Geometry: final body of the model. Coordinates: model frame, mm. Give positions to 0.01 mm unless a question says otherwise; leave off trailing zeros. Write each loop counter-clockwise with the first axis right and the second up, starting at its lowest first coordinate (ties: lowest second). Pieces come first, ordered by that corner, then holes. Notation, with made-up numbers: M -18,-17 L 30,-17 A28 cw 30,20 Z; hole C -2.5,0 d9. An arc over 180 degrees is marked long. Use a Markdown table: item, result. Add a question column.
(1) Cut plane B-B (x = -423.5). Output: boundary loops of the cut face in (y, z).
(2) Cut plane A-A (y = -565). Output: boundary loops of the cut face in (x, z).
(3) Pin query (flat end, axial travel): pin 1 Ø14 at (y, z) = (-533, 39.5) entering from +X; pin 2 Ø10 at (x, z) = (554, 38) entering from +Y; pin 3 Ø6.5 at (x, z) = (-301.5, 7.5) entering from -Y. Return the tip coordinate at first contact, or that it passes through.
(4) Material intervals for L1, parallel to Y at x = 155, z = 35; L2, parallel to X at y = -472, z = 11.5, sorted ascending.
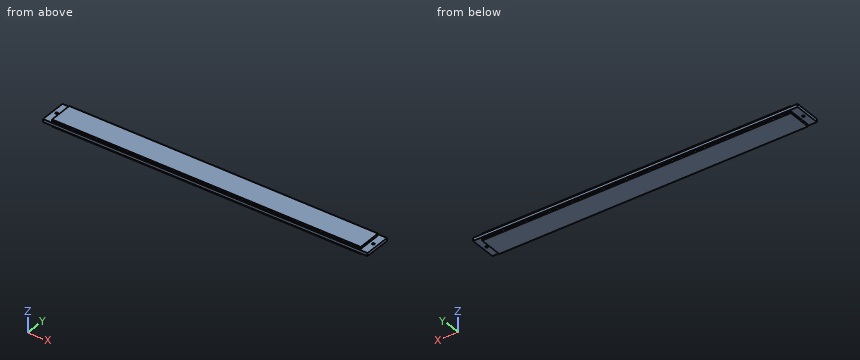
```python
from build123d import *

# Parameters (mm, degrees)
F0_W     = 2082.8
F0_H     = 171.45
F1_DEPTH = 44.45
F2_W     = 1981.2
F2_H     = 9.525
F3_DEPTH = 12.7
F4_W     = 1981.2
F4_H     = 9.525
F5_DEPTH = 12.7
F6_W     = 12.7
F6_H     = 12.7
F7_DEPTH = 31.751


with BuildPart() as f1:
    # F0 (on Top) → F1 (new body)
    with BuildSketch(Plane.XY):
        with Locations((80.949743, -507.08936)):
            Rectangle(F0_W, F0_H)
    extrude(amount=F1_DEPTH)

    # F2 (on face) → F3 (cut)
    with BuildSketch(Plane(origin=(0, 0, 0), x_dir=(1, 0, 0), z_dir=(0, 0, -1))):
        Polygon((-960.450257, 592.81436), (-960.450257, 421.36436), (-909.650257, 421.36436), (-909.650257, 430.88936), (-909.650257, 583.28936), (-909.650257, 592.81436), align=None)
        with Locations((80.949743, 426.12686)):
            Rectangle(F2_W, F2_H)
        Polygon((1071.549743, 430.88936), (1071.549743, 421.36436), (1122.349743, 421.36436), (1122.349743, 592.81436), (1071.549743, 592.81436), (1071.549743, 583.28936), align=None)
        with Locations((80.949743, 588.05186)):
            Rectangle(F2_W, F2_H)
    extrude(amount=-F3_DEPTH, mode=Mode.SUBTRACT)

    # F4 (on face) → F5 (cut)
    with BuildSketch(Plane.XY.offset(44.45)):
        Polygon((1122.349743, -421.36436), (1071.549743, -421.36436), (1071.549743, -430.88936), (1071.549743, -583.28936), (1071.549743, -592.81436), (1122.349743, -592.81436), align=None)
        with Locations((80.949743, -426.12686)):
            Rectangle(F4_W, F4_H)
        Polygon((-909.650257, -430.88936), (-909.650257, -421.36436), (-960.450257, -421.36436), (-960.450257, -592.81436), (-909.650257, -592.81436), (-909.650257, -583.28936), align=None)
        with Locations((80.949743, -588.05186)):
            Rectangle(F4_W, F4_H)
    extrude(amount=-F5_DEPTH, mode=Mode.SUBTRACT)

    # F6 (on face) → F7 (cut, through all)
    with BuildSketch(Plane(origin=(0, 0, 12.7), x_dir=(1, 0, 0), z_dir=(0, 0, -1))):
        with Locations((-935.050257, 507.08936)):
            Rectangle(F6_W, F6_H)
        with Locations((1096.949743, 507.08936)):
            Rectangle(F6_W, F6_H)
    extrude(amount=-F7_DEPTH, mode=Mode.SUBTRACT)


solid = f1.part
```
Answer list:
| question | item | result |
|---|---|---|
| 1 | outline | M -592.81,12.7 L -583.29,12.7 L -583.29,0 L -430.89,0 L -430.89,12.7 L -421.36,12.7 L -421.36,31.75 L -430.89,31.75 L -430.89,44.45 L -583.29,44.45 L -583.29,31.75 L -592.81,31.75 Z |
| 2 | outline | M -960.45,12.7 L -909.65,12.7 L -909.65,0 L 1071.55,0 L 1071.55,12.7 L 1122.35,12.7 L 1122.35,31.75 L 1071.55,31.75 L 1071.55,44.45 L -909.65,44.45 L -909.65,31.75 L -960.45,31.75 Z |
| 3 | pin 1 | x = 1071.55 |
| 3 | pin 2 | y = -430.89 |
| 3 | pin 3 | y = -583.29 |
| 4 | L1 | -583.29 to -430.89 |
| 4 | L2 | -909.65 to 1071.55 |
